Verification items for the finished model (mm, model axes). Round coordinates to 2 decimals unless told otherwise and drop trailing zeros. Loops run counter-clockwise (first coordinate to the right, second up) from the corner with the lowest first, then second, coordinate; pieces in that order, holes last. Notation, with made-up numbers: M -36,-18.5 L -7,-18.5 A12 cw -7,-11.5 Z; hole C -23,28 d5. An arc over 180 degrees is marked long. Write item = value, one per line. Start each with the question number.
from build123d import *

# Parameters (mm, degrees)
BOSS_EXTRUDE1_DEPTH = 2.5
SKETCH2_R           = 1.7
SKETCH2_R_2         = 7.5
CUT_EXTRUDE1_DEPTH  = 142.178079035


with BuildPart() as part:
    # Sketch1 → Boss-Extrude1 (new body)
    with BuildSketch(Plane(origin=(0, 0, 0), x_dir=(1, 0, 0), z_dir=(0, 1, 0))):
        with BuildLine():
            Line((10, 0), (120, 0))
            ThreePointArc((120, 0), (127.071067812, 2.928932188), (130, 10))
            Line((130, 10), (130, 45))
            ThreePointArc((130, 45), (127.071067812, 52.071067812), (120, 55))
            Line((120, 55), (10, 55))
            ThreePointArc((10, 55), (2.928932188, 52.071067812), (0, 45))
            Line((0, 45), (0, 10))
            ThreePointArc((0, 10), (2.928932188, 2.928932188), (10, 0))
        make_face()
    extrude(amount=BOSS_EXTRUDE1_DEPTH)

    # Sketch2 → Cut-Extrude1 (cut, through all)
    with BuildSketch(Plane(origin=(0, 2.5, 0), x_dir=(1, 0, 0), z_dir=(0, 1, 0))):
        with Locations(Location((14, 5, 0), (0, 0, 270))):
            Circle(SKETCH2_R)
        with Locations(Location((14, 50, 0), (0, 0, 270))):
            Circle(SKETCH2_R)
        with Locations(Location((116, 5, 0), (0, 0, 90))):
            Circle(SKETCH2_R)
        with Locations(Location((116, 50, 0), (0, 0, 90))):
            Circle(SKETCH2_R)
        with Locations(Location((14, 27.5, 0), (0, 0, 270))):
            Circle(SKETCH2_R_2)
        with Locations(Location((116, 27.5, 0), (0, 0, 90))):
            Circle(SKETCH2_R_2)
        with Locations(Location((65, 35, 0), (0, 0, 270))):
            Circle(SKETCH2_R)
        with Locations(Location((65, 20, 0), (0, 0, 90))):
            Circle(SKETCH2_R)
    extrude(amount=-CUT_EXTRUDE1_DEPTH, mode=Mode.SUBTRACT)


solid = part.part
1. Section check A-A, the plane x = 116. Enter the section's corners in (y, z), and give its area (3 significant figures).
2. Section check C-C, the plane x = 65. Enter the section's corners in (y, z).
3. Section check D-D, the plane z = -5. Enter the section's corners in (x, y).
4. Section check B-B, the plane y = 1.5. Give the number of separate pieces and of enclosed holes in the cut face, and give its area (3 significant figures).
5. Thickness scan on line 1 (X direction, y = 1.95, z = -27.5); line 2 (Z direction, x = 116, y = 0.6); line 3 (X direction, y = 1.1, z = -50). Record the ranges inside material, lowest first.
6. Mould release check, pull along Z, two halves, no side actions. Record for faces 1 (the flat face through (64, 1, 0)), 2 (the flat face through (64, 2.5, -28)), 3 (the cylindrical face through (63.567, 1.268, -20.914)): pulls with the +Z half, pulls with the -Z half, needs draft (parallel to the pull), parting line crosses it, or undercut.
7. Gauge pin test, flat end, axial feed: P1, Ø5.5, axis at x = 14, z = -50, coming from the +Y side. Record the tip position at first contact, or that the pin passes through.
Computed values:
q1.outline = M 0,-55 L 2.5,-55 L 2.5,-51.7 L 0,-51.7 Z; M 0,-48.3 L 2.5,-48.3 L 2.5,-35 L 0,-35 Z; M 0,-20 L 2.5,-20 L 2.5,-6.7 L 0,-6.7 Z; M 0,-3.3 L 2.5,-3.3 L 2.5,0 L 0,0 Z
q1.area = 83.0 mm2
q2.outline = M 0,-55 L 2.5,-55 L 2.5,-36.7 L 0,-36.7 Z; M 0,-33.3 L 2.5,-33.3 L 2.5,-21.7 L 0,-21.7 Z; M 0,-18.3 L 2.5,-18.3 L 2.5,0 L 0,0 Z
q3.outline = M 1.34,0 L 12.3,0 L 12.3,2.5 L 1.34,2.5 Z; M 15.7,0 L 114.3,0 L 114.3,2.5 L 15.7,2.5 Z; M 117.7,0 L 128.66,0 L 128.66,2.5 L 117.7,2.5 Z
q4.separate_pieces = 1
q4.enclosed_holes = 8
q4.area = 6,660 mm2
q5.line_1 = 0 to 6.5, 21.5 to 108.5, 123.5 to 130
q5.line_2 = -55 to -51.7, -48.3 to -35, -20 to -6.7, -3.3 to 0
q5.line_3 = 1.34 to 12.3, 15.7 to 114.3, 117.7 to 128.66
q6.face_1 = pulls with the +Z half
q6.face_2 = needs draft
q6.face_3 = undercut
q7.P1 = 2.5
